from build123d import *

# Parameters (mm, degrees)
F0_W     = 914.4
F0_H     = 1181.1
F1_DEPTH = 25.4
F2_W     = 914.4
F2_H     = 1181.1
F2_W_2   = 863.6
F2_H_2   = 25.4
F3_DEPTH = 228.6


with BuildPart() as f1:
    # F0 (on Right) → F1 (new body)
    with BuildSketch(Plane.YZ):
        Rectangle(F0_W, F0_H)
    extrude(amount=F1_DEPTH)

    # F2 (on face) → F3 (join)
    with BuildSketch(Plane(origin=(0, 0, 0), x_dir=(0, -1, 0), z_dir=(-1, 0, 0))):
        Rectangle(F2_W, F2_H)
        Polygon((-431.8, 565.15), (431.8, 565.15), (431.8, 301.625), (431.8, 276.225), (431.8, 12.7), (431.8, -12.7), (431.8, -276.225), (431.8, -301.625), (431.8, -565.15), (-431.8, -565.15), (-431.8, -301.625), (-431.8, -276.225), (-431.8, -12.7), (-431.8, 12.7), (-431.8, 276.225), (-431.8, 301.625), align=None, mode=Mode.SUBTRACT)
        with Locations((0, 288.925)):
            Rectangle(F2_W_2, F2_H_2)
        Rectangle(F2_W_2, F2_H_2)
        with Locations((0, -288.925)):
            Rectangle(F2_W_2, F2_H_2)
    extrude(amount=F3_DEPTH)


solid = f1.part
Input: part model. Units: mm. Frame: model coordinates. Coordinates: 2 decimals unless noted, no trailing zeros. Loops run counter-clockwise (first coordinate to the right, second up) from the corner with the lowest first, then second, coordinate; pieces in that order, holes last. Notation, with made-up numbers: (-26, -26.5) -> (-9, -26.5) arc R21 ccw to (-9, -5.5) -> close; hole circle Ø4 at (74.5, 48.5). An arc over 180 degrees is marked (long way). Write item = value, one per line. Start each with the question number.
Item 1: Cut plane A-A, the plane x = -206. Return loops of the section in (y, z) (3 decimals), plus the area to 3 significant figures.
Item 2: Cut plane B-B, the plane y = -318.5. Return loops of the section in (x, z) (3 decimals).
Item 3: Material intervals for line 1 (Z direction, x = -38, y = 337.5) (3 decimals); line 2 (Y direction, x = -39, z = -437.5); line 3 (X direction, y = 169, z = -540), sorted ascending.
Item 4: Mould query, pull axis Y, two halves, no side actions, for faces 1 (the face through (-100, -457.2, -8)), 2 (the face through (25.4, -6, 8)), 3 (the face through (-113, 431.8, -146)). Classes: pulls with the +Y half, pulls with the -Y half, needs draft (parallel to the pull), parting line crosses it, or undercut.
Item 5: First-contact query: P1, Ø5, axis at y = -19, z = -78, coming from the -X side. Flat tip, straight axial feed; report the tip coordinate or a pass-through.
Item 6: Cut plane C-C, the plane z = -73. Return loops of the section in (x, y), plus the area to 3 significant figures.
Ans:
q1.outline = (-457.2, -590.55) -> (457.2, -590.55) -> (457.2, 590.55) -> (-457.2, 590.55) -> close; hole (-431.8, -565.15) -> (431.8, -565.15) -> (431.8, -301.625) -> (-431.8, -301.625) -> close; hole (-431.8, -276.225) -> (431.8, -276.225) -> (431.8, -12.7) -> (-431.8, -12.7) -> close; hole (-431.8, 12.7) -> (431.8, 12.7) -> (431.8, 276.225) -> (-431.8, 276.225) -> close; hole (-431.8, 301.625) -> (431.8, 301.625) -> (431.8, 565.15) -> (-431.8, 565.15) -> close
q1.area = 170,000 mm²
q2.outline = (-228.6, -590.55) -> (25.4, -590.55) -> (25.4, 590.55) -> (-228.6, 590.55) -> (-228.6, 565.15) -> (0, 565.15) -> (0, 301.625) -> (-228.6, 301.625) -> (-228.6, 276.225) -> (0, 276.225) -> (0, 12.7) -> (-228.6, 12.7) -> (-228.6, -12.7) -> (0, -12.7) -> (0, -276.225) -> (-228.6, -276.225) -> (-228.6, -301.625) -> (0, -301.625) -> (0, -565.15) -> (-228.6, -565.15) -> close
q3.line_1 = -590.55 to -565.15, -301.625 to -276.225, -12.7 to 12.7, 276.225 to 301.625, 565.15 to 590.55
q3.line_2 = -457.2 to -431.8, 431.8 to 457.2
q3.line_3 = 0 to 25.4
q4.face_1 = pulls with the -Y half
q4.face_2 = needs draft
q4.face_3 = undercut
q5.P1 = 0
q6.outline = (-228.6, -457.2) -> (25.4, -457.2) -> (25.4, 457.2) -> (-228.6, 457.2) -> (-228.6, 431.8) -> (0, 431.8) -> (0, -431.8) -> (-228.6, -431.8) -> close
q6.area = 34,800 mm²
